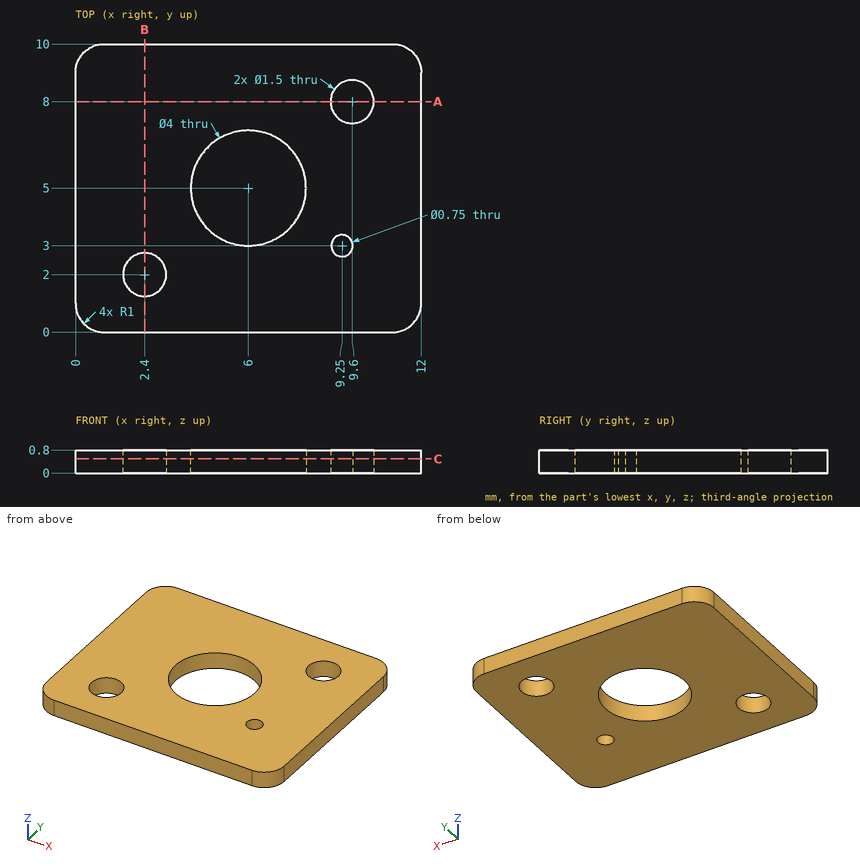
Design review of the part shown in the three views and the two pictorial views. Dimensions are in mm from the part's minimum x, y and z. Round coordinates to 2 decimals unless told otherwise and drop trailing zeros. Write each loop counter-clockwise with the first axis right and the second up, starting at its lowest first coordinate (ties: lowest second). Pieces come first, ordered by that corner, then holes.
Item 1: We need section B-B on x = 2.4. Write out the cut boundary in (y, z).
Item 2: For probe 1 along Y at (x, z) = (6, 0.45); probe 2 along Y at (x, z) = (2.4, 0.3); probe 3 along X at (y, z) = (6.25, 0.65), list the stretches that pass through material, from the lowest coordinate up.
Item 3: We need section C-C on z = 0.5. Write out the cut boundary in (x, y) (3 decimals), and give its area (3 significant figures).
Item 4: We need section A-A on y = 8. Write out the cut boundary in (x, z), and give its area (3 significant figures).
Returned:
1. outline: (0, 0) - (1.25, 0) - (1.25, 0.8) - (0, 0.8) - close; (2.75, 0) - (10, 0) - (10, 0.8) - (2.75, 0.8) - close
2. probe 1: y = 0 to 3, 7 to 10
2. probe 2: y = 0 to 1.25, 2.75 to 10
2. probe 3: x = 0 to 4.44, 7.56 to 12
3. outline: (0, 1) arc R1 ccw to (1, 0) - (11, 0) arc R1 ccw to (12, 1) - (12, 9) arc R1 ccw to (11, 10) - (1, 10) arc R1 ccw to (0, 9) - close; hole circle Ø1.5 at (2.4, 2); hole circle Ø4 at (6, 5); hole circle Ø1.5 at (9.6, 8); hole circle Ø0.75 at (9.25, 3)
3. area: 103 mm2
4. outline: (0, 0) - (8.85, 0) - (8.85, 0.8) - (0, 0.8) - close; (10.35, 0) - (12, 0) - (12, 0.8) - (10.35, 0.8) - close
4. area: 8.40 mm2
